from build123d import *

# Parameters (mm, degrees)
F0_W           = 106
F0_H           = 174
F1_DEPTH       = 4
F2_R           = 2
F3_T1_DEPTH    = 7
F3_S5_W        = 2
F3_S5_H        = 2
F3_T6_DEPTH    = 2
F3_S11_W       = 2
F3_S11_H       = 2
F3_T12_DEPTH   = 2
F3_S17_W       = 2
F3_S17_H       = 2
F3_T18_DEPTH   = 2
F3_S23_W       = 2
F3_S23_H       = 2
F3_T24_DEPTH   = 2
F5_D           = 4.1
F5_DEPTH       = 40
F5_CSINK_D     = 8
F5_CSINK_ANGLE = 90
F5_TIP         = 1.231764269


# Not quite as in the source:
# - a fillet or chamfer that OpenCascade refuses, or shapes differently, is made with other operations: its cross-section is extruded or revolved along the edge and cut away or added


with BuildPart() as f1:
    # F0 (on Top) → F1 (new body)
    with BuildSketch(Plane.XY):
        with Locations((53, 87)):
            Rectangle(F0_W, F0_H)
    extrude(amount=F1_DEPTH)

    # F2
    f2_edges = [f1.edges().sort_by_distance(p)[0] for p in [
        (53, 0, 4),
        (0, 87, 4),
        (106, 87, 4),
        (53, 174, 4),
    ]]
    fillet(f2_edges, radius=F2_R)

    # F3: fillet of radius 2 on 4 edges, made by hand

    # F3_s2 → F3_t1 (cut)
    with BuildSketch(Plane.XY.offset(-5)):
        with BuildLine():
            ThreePointArc((104, 0), (105.4142135624, 0.5857864376), (106, 2))
            Line((106, 2), (106, 0))
            Line((106, 0), (104, 0))
        make_face()
        with BuildLine():
            ThreePointArc((0, 2), (0.5857864376, 0.5857864376), (2, 0))
            Line((2, 0), (0, 0))
            Line((0, 0), (0, 2))
        make_face()
        with BuildLine():
            ThreePointArc((0, 172), (0.5857864376, 173.4142135624), (2, 174))
            Line((2, 174), (0, 174))
            Line((0, 174), (0, 172))
        make_face()
        with BuildLine():
            ThreePointArc((104, 174), (105.4142135624, 173.4142135624), (106, 172))
            Line((106, 172), (106, 174))
            Line((106, 174), (104, 174))
        make_face()
    extrude(amount=F3_T1_DEPTH, mode=Mode.SUBTRACT)


with BuildPart() as f3_tool4:
    # F3_s5 → F3_t6 (new body)
    with BuildSketch(Plane.XZ.offset(-172)):
        with Locations((105, 3)):
            Rectangle(F3_S5_W, F3_S5_H)
    extrude(amount=-F3_T6_DEPTH)

    # F3_s7 → F3_t8 (revolve, cut)
    with BuildSketch(Plane(origin=(104, 172, 2), x_dir=(-0.7071067812, 0, -0.7071067812), z_dir=(0.7071067812, 0, -0.7071067812))):
        with BuildLine():
            ThreePointArc((0, -2), (2, 0), (0, 2))
            Line((0, 2), (0, -2))
        make_face()
    revolve(axis=Axis((104, 172, 2), (0, 1, 0)), mode=Mode.SUBTRACT)


with BuildPart() as f1_1:
    add(f1.part)

    # F3_t3: cut F3_tool4
    add(f3_tool4.part, mode=Mode.SUBTRACT)


with BuildPart() as f3_tool10:
    # F3_s11 → F3_t12 (new body)
    with BuildSketch(Plane.YZ.offset(2)):
        with Locations((173, 3)):
            Rectangle(F3_S11_W, F3_S11_H)
    extrude(amount=-F3_T12_DEPTH)

    # F3_s13 → F3_t14 (revolve, cut)
    with BuildSketch(Plane(origin=(2, 172, 2), x_dir=(0, -0.7071067812, -0.7071067812), z_dir=(0, 0.7071067812, -0.7071067812))):
        with BuildLine():
            ThreePointArc((0, -2), (2, 0), (0, 2))
            Line((0, 2), (0, -2))
        make_face()
    revolve(axis=Axis((2, 172, 2), (-1, 0, 0)), mode=Mode.SUBTRACT)


with BuildPart() as f1_2:
    add(f1_1.part)

    # F3_t9: cut F3_tool10
    add(f3_tool10.part, mode=Mode.SUBTRACT)


with BuildPart() as f3_tool16:
    # F3_s17 → F3_t18 (new body)
    with BuildSketch(Plane.YZ.offset(2)):
        with Locations((1, 3)):
            Rectangle(F3_S17_W, F3_S17_H)
    extrude(amount=-F3_T18_DEPTH)

    # F3_s19 → F3_t20 (revolve, cut)
    with BuildSketch(Plane(origin=(2, 2, 2), x_dir=(0, 0.7071067812, -0.7071067812), z_dir=(0, 0.7071067812, 0.7071067812))):
        with BuildLine():
            ThreePointArc((0, -2), (2, 0), (0, 2))
            Line((0, 2), (0, -2))
        make_face()
    revolve(axis=Axis((2, 2, 2), (-1, 0, 0)), mode=Mode.SUBTRACT)


with BuildPart() as f1_3:
    add(f1_2.part)

    # F3_t15: cut F3_tool16
    add(f3_tool16.part, mode=Mode.SUBTRACT)


with BuildPart() as f3_tool22:
    # F3_s23 → F3_t24 (new body)
    with BuildSketch(Plane.XZ.offset(-2)):
        with Locations((105, 3)):
            Rectangle(F3_S23_W, F3_S23_H)
    extrude(amount=F3_T24_DEPTH)

    # F3_s25 → F3_t26 (revolve, cut)
    with BuildSketch(Plane(origin=(104, 2, 2), x_dir=(-0.7071067812, 0, -0.7071067812), z_dir=(-0.7071067812, 0, 0.7071067812))):
        with BuildLine():
            ThreePointArc((0, -2), (2, 0), (0, 2))
            Line((0, 2), (0, -2))
        make_face()
    revolve(axis=Axis((104, 2, 2), (0, -1, 0)), mode=Mode.SUBTRACT)


with BuildPart() as f1_4:
    add(f1_3.part)

    # F3_t21: cut F3_tool22
    add(f3_tool22.part, mode=Mode.SUBTRACT)

    # F5
    with Locations(Plane.XY.offset(4)):
        with Locations((10, 164), (10, 10), (96, 164), (96, 10)):
            CounterSinkHole(F5_D / 2, F5_CSINK_D / 2, depth=F5_DEPTH, counter_sink_angle=F5_CSINK_ANGLE)
            with Locations((0, 0, -(F5_DEPTH + F5_TIP / 2))):  # 118° drill point
                Cone(0, F5_D / 2, F5_TIP, mode=Mode.SUBTRACT)


solid = f1_4.part
For this review, take the finished solid that the model builds, in its own axes (mm). Round coordinates to 2 decimals unless told otherwise and drop trailing zeros. Write each loop counter-clockwise with the first axis right and the second up, starting at its lowest first coordinate (ties: lowest second). Pieces come first, ordered by that corner, then holes. Notation, with made-up numbers: (67, -9.75) - (124, -9.75) arc R21 cw to (124, 7.25) - close; hole circle Ø7 at (74, 42). An arc over 180 degrees is marked (long way). Write item = value, one per line. Start each with the question number.
1. Wall thickness on L1, parallel to X at y = 10, z = 1.5; L2, parallel to Y at x = 10, z = 0.7; L3, parallel to X at y = 34, z = 2.3: over which ranges is each line inside the solid? List them lowest first.
2. Draft analysis for pull direction X (two halves, no side actions). For faces 1 (the face through (52, 88, 4)), 2 (the face through (10.267, 166.033, 1.011)), state which applies: released by +X, released by -X, zero draft, split by the parting line, or undercut.
3. Consider section B-B on y = 164. State the section outline as (x, z) points.
4. Consider section A-A on x = 96. State the section outline as (y, z) points.
5. For pin 1 Ø4.5 at (x, y) = (10, 164) entering from +Z; pin 2 Ø6.5 at (x, y) = (10, 10) entering from +Z, all flat-tipped, find the tip position at first contact; note any pin that passes through.
Evaluation:
q1.L1 = 0 to 7.95, 12.05 to 93.95, 98.05 to 106
q1.L2 = 0 to 7.95, 12.05 to 161.95, 166.05 to 174
q1.L3 = 0.02 to 105.98
q2.face_1 = zero draft
q2.face_2 = undercut
q3.outline = (0, 0) - (7.95, 0) - (7.95, 2.05) - (6, 4) - (2, 4) arc R2 ccw to (0, 2) - close; (12.05, 0) - (93.95, 0) - (93.95, 2.05) - (92, 4) - (14, 4) - (12.05, 2.05) - close; (98.05, 0) - (106, 0) - (106, 2) arc R2 ccw to (104, 4) - (100, 4) - (98.05, 2.05) - close
q4.outline = (0, 0) - (7.95, 0) - (7.95, 2.05) - (6, 4) - (2, 4) arc R2 ccw to (0, 2) - close; (12.05, 0) - (161.95, 0) - (161.95, 2.05) - (160, 4) - (14, 4) - (12.05, 2.05) - close; (166.05, 0) - (174, 0) - (174, 2) arc R2 ccw to (172, 4) - (168, 4) - (166.05, 2.05) - close
q5.pin_1 = 2.25
q5.pin_2 = 3.25
